```python
from build123d import *

# Parameters (mm, degrees)
SKETCH1_R           = 3
BOSS_EXTRUDE1_DEPTH = 10
SKETCH2_R           = 1.6
CUT_EXTRUDE1_DEPTH  = 10
CHAMFER1_SIZE       = 0.5


with BuildPart() as part:
    # Sketch1 → Boss-Extrude1 (new body)
    with BuildSketch(Plane(origin=(0, 0, 0), x_dir=(1, 0, 0), z_dir=(0, 1, 0))):
        Circle(SKETCH1_R)
    extrude(amount=BOSS_EXTRUDE1_DEPTH)

    # Sketch2 → Cut-Extrude1 (cut)
    with BuildSketch(Plane(origin=(0, 10, 0), x_dir=(1, 0, 0), z_dir=(0, 1, 0))):
        Circle(SKETCH2_R)
    extrude(amount=-CUT_EXTRUDE1_DEPTH, mode=Mode.SUBTRACT)

    # Chamfer1
    chamfer1_edges = [part.edges().sort_by_distance(p)[0] for p in [
        (-3, 0, 0),
        (-3, 10, 0),
    ]]
    chamfer(chamfer1_edges, length=CHAMFER1_SIZE)


solid = part.part
```
Can you work these out from the model? Positions are in its coordinate system, mm. Give positions to 0.01 mm unless a question says otherwise; leave off trailing zeros. Write each loop counter-clockwise with the first axis right and the second up, starting at its lowest first coordinate (ties: lowest second). Pieces come first, ordered by that corner, then holes. Notation, with made-up numbers: (-6, 53.25) -> (-1, 53.25) arc R19 cw to (-1, 57.25) -> close; hole circle Ø9 at (-33, 35.25). An arc over 180 degrees is marked (long way). One line per item, written item: value.
Q1. We'd pull the mould along X, two halves only. Please class faces 1 (the face through (-1.27, 5.07, 0.97)), 2 (the face through (-3, 5, 0)), 3 (the face through (0, 0, 2)): +X half, -X half, draft (parallel to the pull), parting line (faces both ways), or undercut.
Results found:
face 1: undercut
face 2: parting line
face 3: draft
Q2. Imagine slicing it at C-C on y = 4.75. Please give me the cut outline in (x, z).
Results found:
outline: circle Ø6 at (0, 0); hole circle Ø3.2 at (0, 0)
Q3. Please list where these lines run through material, in increasing order: line 1 (X direction, y = 6.5, z = 0); line 2 (Z direction, x = -1.25, y = 4.75). Write a range as [from, to].
Results found:
line 1: x = [-3, -1.6], [1.6, 3]
line 2: z = [-2.73, -1], [1, 2.73]
Q4. Imagine slicing it at B-B on z = 0. Please give me the cut outline in (x, y).
Results found:
outline: (-3, 0.5) -> (-2.5, 0) -> (-1.6, 0) -> (-1.6, 10) -> (-2.5, 10) -> (-3, 9.5) -> close; (1.6, 0) -> (2.5, 0) -> (3, 0.5) -> (3, 9.5) -> (2.5, 10) -> (1.6, 10) -> close
Q5. Imagine slicing it at A-A on x = 0. Please give me the cut outline in (y, z), and give its area (3 significant figures).
Results found:
outline: (0, -2.5) -> (0.5, -3) -> (9.5, -3) -> (10, -2.5) -> (10, -1.6) -> (0, -1.6) -> close; (0, 1.6) -> (10, 1.6) -> (10, 2.5) -> (9.5, 3) -> (0.5, 3) -> (0, 2.5) -> close
area: 27.5 mm^2
